Source: CAD feature listing. Evaluate the final solid. Frame: model axes, mm. A direction names the side the tool comes from. Give positions to 0.01 mm unless a question says otherwise; leave off trailing zeros. Order: outer loops, then holes, each group sorted by start corner. A loop starts at its lowest first (then second) coordinate and runs counter-clockwise, first axis right, second up.
from build123d import *

# Parameters (mm, degrees)
CROQUIS1_R              = 13
SALIENTE_EXTRUIR1_DEPTH = 3
CROQUIS2_W              = 50
CROQUIS2_H              = 6
SALIENTE_EXTRUIR2_DEPTH = 9
CROQUIS3_W              = 50
CROQUIS3_H              = 6
SALIENTE_EXTRUIR3_DEPTH = 107
CROQUIS4_W              = 50
CROQUIS4_H              = 6
SALIENTE_EXTRUIR4_DEPTH = 6
CROQUIS5_R              = 2.5
CORTAR_EXTRUIR1_DEPTH   = 116.021737076
CROQUIS6_W              = 50
CROQUIS6_H              = 6
SALIENTE_EXTRUIR5_DEPTH = 18
CROQUIS7_W              = 50
CROQUIS7_H              = 6
SALIENTE_EXTRUIR6_DEPTH = 18
CROQUIS8_R              = 3
SALIENTE_EXTRUIR7_DEPTH = 10
SALIENTE_EXTRUIR8_DEPTH = 3


with BuildPart() as part:
    # Croquis1 → Saliente-Extruir1 (new, symmetric)
    with BuildSketch(Plane.XY):
        with BuildLine():
            Line((25, -9), (-25, -9))
            Line((-25, -9), (-25, 9))
            ThreePointArc((-25, 9), (0, 34), (25, 9))
            Line((25, 9), (25, -9))
        make_face()
        with Locations((0, 9)):
            Circle(CROQUIS1_R, mode=Mode.SUBTRACT)
    extrude(amount=SALIENTE_EXTRUIR1_DEPTH, both=True)

    # Croquis2 → Saliente-Extruir2 (add)
    with BuildSketch(Plane.XZ.offset(9)):
        Rectangle(CROQUIS2_W, CROQUIS2_H)
    extrude(amount=SALIENTE_EXTRUIR2_DEPTH)



with BuildPart() as body_2:
    # Croquis3 → Saliente-Extruir3 (new body)
    with BuildSketch(Plane.XY.offset(3)):
        with Locations((0, -15)):
            Rectangle(CROQUIS3_W, CROQUIS3_H)
    extrude(amount=SALIENTE_EXTRUIR3_DEPTH)


with BuildPart() as part_1:
    add(part.part)

    add(body_2.part)  # Saliente-Extruir4 merges body 2
    # Croquis4 → Saliente-Extruir4 (add)
    with BuildSketch(Plane(origin=(0, 0, 3), x_dir=(-1, 0, 0), z_dir=(0, 0, -1))):
        with Locations((0, -15)):
            Rectangle(CROQUIS4_W, CROQUIS4_H)
    extrude(amount=SALIENTE_EXTRUIR4_DEPTH)

    # Croquis5 → Cortar-Extruir1 (cut, through all)
    with BuildSketch(Plane.XY.offset(3)):
        with Locations((12.727922061, 21.727922061)):
            Circle(CROQUIS5_R)
        with Locations((12.727922061, -3.727922061)):
            Circle(CROQUIS5_R)
        with Locations((-12.727922061, -3.727922061)):
            Circle(CROQUIS5_R)
        with Locations((-12.727922061, 21.727922061)):
            Circle(CROQUIS5_R)
    extrude(amount=-CORTAR_EXTRUIR1_DEPTH, mode=Mode.SUBTRACT)

    # Croquis6 → Saliente-Extruir5 (add)
    with BuildSketch(Plane.XY.offset(110)):
        with Locations((0, -15)):
            Rectangle(CROQUIS6_W, CROQUIS6_H)
    extrude(amount=SALIENTE_EXTRUIR5_DEPTH)

    # Croquis7 → Saliente-Extruir6 (add)
    with BuildSketch(Plane(origin=(0, 0, -3), x_dir=(-1, 0, 0), z_dir=(0, 0, -1))):
        with Locations((0, -15)):
            Rectangle(CROQUIS7_W, CROQUIS7_H)
    extrude(amount=SALIENTE_EXTRUIR6_DEPTH)

    # Croquis8 → Saliente-Extruir7 (add)
    with BuildSketch(Plane(origin=(20, 0, 0), x_dir=(0, 0, -1), z_dir=(1, 0, 0))):
        with BuildLine():
            Line((3, -4), (3, -12))
            Line((3, -12), (13, -12))
            Line((13, -12), (13, -4))
            ThreePointArc((13, -4), (8, 1), (3, -4))
        make_face()
        with Locations((8, -4)):
            Circle(CROQUIS8_R, mode=Mode.SUBTRACT)
    saliente_extruir7 = extrude(amount=-SALIENTE_EXTRUIR7_DEPTH)

    # Simetría1: Saliente-Extruir7 across plane
    add(saliente_extruir7.mirror(Plane(origin=(0, 0, 53.5), x_dir=(1, 0, 0), z_dir=(0, 0, -1))))

    # Croquis9 → Saliente-Extruir8 (add)
    with BuildSketch(Plane(origin=(25, 0, 0), x_dir=(0, 0, -1), z_dir=(1, 0, 0))):
        Polygon((-128, -18), (21, -18), (21, -12), (3, -12), (-128, -12), align=None)
    extrude(amount=SALIENTE_EXTRUIR8_DEPTH)


solid = part_1.part
1) Section query C-C on z = 115. Output: boundary loops of the cut face in (x, y), and give its area (3 significant figures).
Checks:
outline: (-25, -18) - (28, -18) - (28, -12) - (20, -12) - (20, -7) - (10, -7) - (10, -12) - (-25, -12) - close; (10, -1) - (20, -1) - (20, 1) - (10, 1) - close
area: 388 mm2
2) Section query A-A on y = 4. Output: boundary loops of the cut face in (x, z).
Checks:
outline: (-25, -3) - (-12, -3) - (-12, 3) - (-25, 3) - close; (12, -3) - (25, -3) - (25, 3) - (12, 3) - close
3) Pull-direction query (X, two-part tool) for faces 4 (the face through (10, -7, -9)), 5 (the face through (15, 1, 115)), 6 (the face through (12.186, 19.287, 0.042)), 7 (the face through (-10.343, -2.977, 0.042)); classes: +X half, -X half, draft (parallel to the pull), parting line (faces both ways), or undercut.
Checks:
face 4: -X half
face 5: draft
face 6: undercut
face 7: undercut
4) Section query D-D on x = -19.5. Output: boundary loops of the cut face in (y, z), and give its area (3 significant figures).
Checks:
outline: (-18, -21) - (-12, -21) - (-12, -3) - (24.64, -3) - (24.64, 3) - (-12, 3) - (-12, 128) - (-18, 128) - close
area: 1,110 mm2
5) First-contact query: pin 1 Ø1.1 at (x, y) = (13, -5.5) entering from +Z; pin 2 Ø6.5 at (x, y) = (-12.73, 21.73) entering from -Z; pin 3 Ø3 at (y, z) = (-1.5, 0.5) entering from +X; pin 4 Ø2 at (x, y) = (9, 3.5) entering from -Z. Flat tips, straight axial feed; report the tip coordinate or a pass-through.
Checks:
pin 1: stops at z = 120
pin 2: stops at z = -3
pin 3: stops at x = 25
pin 4: passes through
6) Reachability of faces 1 (the face through (10, -7, 114)), 2 (the face through (15.112, -2.977, 0.042)), 3 (the face through (20, -7, -9)) from +Z, -Z, +X, -X, +Y, -Y: full face, straight path, thin tool, end or side. Return the list, or none.
Checks:
face 1: +Z, -X, +Y
face 2: none
face 3: -Z, +X, +Y
7) Section query B-B on x = 0. Output: boundary loops of the cut face in (y, z).
Checks:
outline: (-18, -21) - (-12, -21) - (-12, -3) - (-4, -3) - (-4, 3) - (-12, 3) - (-12, 128) - (-18, 128) - close; (22, -3) - (34, -3) - (34, 3) - (22, 3) - close
8) Ray query, L1, parallel to Y at x = 0, z = -0.6; L2, parallel to Z at x = 19, y = -11; L3, parallel to Y at x = 15, z = -8. Return the intervals inside material, ascending.
Checks:
L1: y = -18 to -4, 22 to 34
L2: z = -13 to 3, 110 to 120
L3: y = -18 to -7, -1 to 1
